Verification items for the finished model (mm, model axes). Face numbers are marked on the shaded views. A direction names the side the tool comes from. Round coordinates to 2 decimals unless told otherwise and drop trailing zeros. Write each loop counter-clockwise with the first axis right and the second up, starting at its lowest first coordinate (ties: lowest second). Pieces come first, ordered by that corner, then holes. Notation, with made-up numbers: M -14.75,15.5 L 19.25,15.5 A25 cw 19.25,43.5 Z; hole C 25,88.25 d6. An arc over 180 degrees is marked long. One line per question, with ' | ' between items.
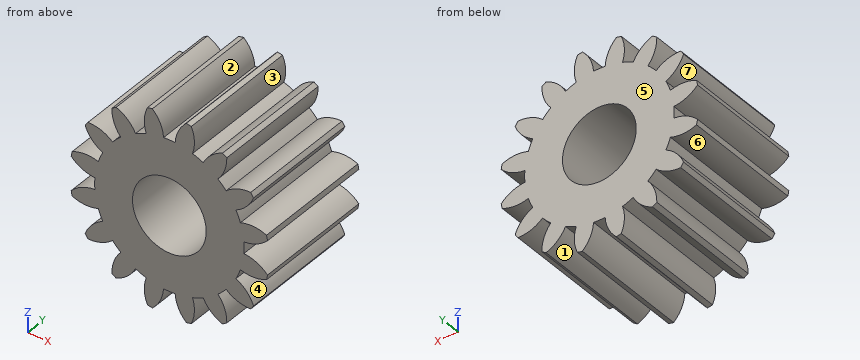
from build123d import *

# Parameters (mm, degrees)
BOSS_EXTRUDE1_DEPTH = 10
SKETCH2_R           = 3
CUT_EXTRUDE1_DEPTH  = 10


with BuildPart() as part:
    # Sketch1 → Boss-Extrude1 (new body)
    with BuildSketch(Plane(origin=(0, 0, 0), x_dir=(1, 0, 0), z_dir=(0, 1, 0))):
        with BuildLine():
            ThreePointArc((-7.982172642, 1.3765609), (-7.105660658, 0.739320543), (-6.05570223, 0.47111199))
            ThreePointArc((-6.05570223, 0.47111199), (-6.074, 0), (-6.05570223, -0.47111199))
            ThreePointArc((-6.05570223, -0.47111199), (-7.105660658, -0.739320543), (-7.982172642, -1.3765609))
            ThreePointArc((-7.982172642, -1.3765609), (-7.944360771, -1.580231608), (-7.901352979, -1.782868784))
            ThreePointArc((-7.901352979, -1.782868784), (-6.84770017, -2.036175492), (-5.775026098, -1.882166189))
            ThreePointArc((-5.775026098, -1.882166189), (-5.61164428, -2.324419168), (-5.414452591, -2.75266764))
            ThreePointArc((-5.414452591, -2.75266764), (-6.281848724, -3.402261728), (-6.847778879, -4.326421665))
            ThreePointArc((-6.847778879, -4.326421665), (-6.73490386, -4.500118887), (-6.617623951, -4.670872857))
            ThreePointArc((-6.617623951, -4.670872857), (-5.547239406, -4.501682267), (-4.615154594, -3.948901628))
            ThreePointArc((-4.615154594, -3.948901628), (-4.294966589, -4.294966589), (-3.948901628, -4.615154594))
            ThreePointArc((-3.948901628, -4.615154594), (-4.501682267, -5.547239406), (-4.670872857, -6.617623951))
            ThreePointArc((-4.670872857, -6.617623951), (-4.500118887, -6.73490386), (-4.326421665, -6.847778879))
            ThreePointArc((-4.326421665, -6.847778879), (-3.402261728, -6.281848724), (-2.75266764, -5.414452591))
            ThreePointArc((-2.75266764, -5.414452591), (-2.324419168, -5.61164428), (-1.882166189, -5.775026098))
            ThreePointArc((-1.882166189, -5.775026098), (-2.036175492, -6.84770017), (-1.782868784, -7.901352979))
            ThreePointArc((-1.782868784, -7.901352979), (-1.580231608, -7.944360771), (-1.3765609, -7.982172642))
            ThreePointArc((-1.3765609, -7.982172642), (-0.739320543, -7.105660658), (-0.47111199, -6.05570223))
            ThreePointArc((-0.47111199, -6.05570223), (0, -6.074), (0.47111199, -6.05570223))
            ThreePointArc((0.47111199, -6.05570223), (0.739320543, -7.105660658), (1.3765609, -7.982172642))
            ThreePointArc((1.3765609, -7.982172642), (1.580231608, -7.944360771), (1.782868784, -7.901352979))
            ThreePointArc((1.782868784, -7.901352979), (2.036175492, -6.84770017), (1.882166189, -5.775026098))
            ThreePointArc((1.882166189, -5.775026098), (2.324419168, -5.61164428), (2.75266764, -5.414452591))
            ThreePointArc((2.75266764, -5.414452591), (3.402261728, -6.281848724), (4.326421665, -6.847778879))
            ThreePointArc((4.326421665, -6.847778879), (4.500118887, -6.73490386), (4.670872857, -6.617623951))
            ThreePointArc((4.670872857, -6.617623951), (4.501682267, -5.547239406), (3.948901628, -4.615154594))
            ThreePointArc((3.948901628, -4.615154594), (4.294966589, -4.294966589), (4.615154594, -3.948901628))
            ThreePointArc((4.615154594, -3.948901628), (5.547239406, -4.501682267), (6.617623951, -4.670872857))
            ThreePointArc((6.617623951, -4.670872857), (6.73490386, -4.500118887), (6.847778879, -4.326421665))
            ThreePointArc((6.847778879, -4.326421665), (6.281848724, -3.402261728), (5.414452591, -2.75266764))
            ThreePointArc((5.414452591, -2.75266764), (5.61164428, -2.324419168), (5.775026098, -1.882166189))
            ThreePointArc((5.775026098, -1.882166189), (6.84770017, -2.036175492), (7.901352979, -1.782868784))
            ThreePointArc((7.901352979, -1.782868784), (7.944360771, -1.580231608), (7.982172642, -1.3765609))
            ThreePointArc((7.982172642, -1.3765609), (7.105660658, -0.739320543), (6.05570223, -0.47111199))
            ThreePointArc((6.05570223, -0.47111199), (6.074, 0), (6.05570223, 0.47111199))
            ThreePointArc((6.05570223, 0.47111199), (7.105660658, 0.739320543), (7.982172642, 1.3765609))
            ThreePointArc((7.982172642, 1.3765609), (7.944360771, 1.580231608), (7.901352979, 1.782868784))
            ThreePointArc((7.901352979, 1.782868784), (6.84770017, 2.036175492), (5.775026098, 1.882166189))
            ThreePointArc((5.775026098, 1.882166189), (5.61164428, 2.324419168), (5.414452591, 2.75266764))
            ThreePointArc((5.414452591, 2.75266764), (6.281848724, 3.402261728), (6.847778879, 4.326421665))
            ThreePointArc((6.847778879, 4.326421665), (6.73490386, 4.500118887), (6.617623951, 4.670872857))
            ThreePointArc((6.617623951, 4.670872857), (5.547239406, 4.501682267), (4.615154594, 3.948901628))
            ThreePointArc((4.615154594, 3.948901628), (4.294966589, 4.294966589), (3.948901628, 4.615154594))
            ThreePointArc((3.948901628, 4.615154594), (4.501682267, 5.547239406), (4.670872857, 6.617623951))
            ThreePointArc((4.670872857, 6.617623951), (4.500118887, 6.73490386), (4.326421665, 6.847778879))
            ThreePointArc((4.326421665, 6.847778879), (3.402261728, 6.281848724), (2.75266764, 5.414452591))
            ThreePointArc((2.75266764, 5.414452591), (2.324419168, 5.61164428), (1.882166189, 5.775026098))
            ThreePointArc((1.882166189, 5.775026098), (2.036175492, 6.84770017), (1.782868784, 7.901352979))
            ThreePointArc((1.782868784, 7.901352979), (1.580231608, 7.944360771), (1.3765609, 7.982172642))
            ThreePointArc((1.3765609, 7.982172642), (0.739320543, 7.105660658), (0.47111199, 6.05570223))
            ThreePointArc((0.47111199, 6.05570223), (0, 6.074), (-0.47111199, 6.05570223))
            ThreePointArc((-0.47111199, 6.05570223), (-0.739320543, 7.105660658), (-1.3765609, 7.982172642))
            ThreePointArc((-1.3765609, 7.982172642), (-1.580231608, 7.944360771), (-1.782868784, 7.901352979))
            ThreePointArc((-1.782868784, 7.901352979), (-2.036175492, 6.84770017), (-1.882166189, 5.775026098))
            ThreePointArc((-1.882166189, 5.775026098), (-2.324419168, 5.61164428), (-2.75266764, 5.414452591))
            ThreePointArc((-2.75266764, 5.414452591), (-3.402261728, 6.281848724), (-4.326421665, 6.847778879))
            ThreePointArc((-4.326421665, 6.847778879), (-4.500118887, 6.73490386), (-4.670872857, 6.617623951))
            ThreePointArc((-4.670872857, 6.617623951), (-4.501682267, 5.547239406), (-3.948901628, 4.615154594))
            ThreePointArc((-3.948901628, 4.615154594), (-4.294966589, 4.294966589), (-4.615154594, 3.948901628))
            ThreePointArc((-4.615154594, 3.948901628), (-5.547239406, 4.501682267), (-6.617623951, 4.670872857))
            ThreePointArc((-6.617623951, 4.670872857), (-6.73490386, 4.500118887), (-6.847778879, 4.326421665))
            ThreePointArc((-6.847778879, 4.326421665), (-6.281848724, 3.402261728), (-5.414452591, 2.75266764))
            ThreePointArc((-5.414452591, 2.75266764), (-5.61164428, 2.324419168), (-5.775026098, 1.882166189))
            ThreePointArc((-5.775026098, 1.882166189), (-6.84770017, 2.036175492), (-7.901352979, 1.782868784))
            ThreePointArc((-7.901352979, 1.782868784), (-7.944360771, 1.580231608), (-7.982172642, 1.3765609))
        make_face()
    extrude(amount=BOSS_EXTRUDE1_DEPTH)

    # Sketch2 → Cut-Extrude1 (cut)
    with BuildSketch(Plane(origin=(0, 10, 0), x_dir=(1, 0, 0), z_dir=(0, 1, 0))):
        Circle(SKETCH2_R)
    extrude(amount=-CUT_EXTRUDE1_DEPTH, mode=Mode.SUBTRACT)


solid = part.part
1. Section check A-A, the plane x = 0. Record the cut outline in (y, z), then the cut area to 3 significant figures.
Results:
outline: M 0,-6.07 L 10,-6.07 L 10,-3 L 0,-3 Z; M 0,3 L 10,3 L 10,6.07 L 0,6.07 Z | area: 61.5 mm2
2. Section check B-B, the plane z = 0. Record the cut outline in (x, y), then the cut area to 3 significant figures.
Results:
outline: M -6.07,0 L -3,0 L -3,10 L -6.07,10 Z; M 3,0 L 6.07,0 L 6.07,10 L 3,10 Z | area: 61.5 mm2
3. Go/stop test with flat-tipped pins: P1, Ø3, axis at y = 4.5, z = -5.5, coming from the -X side; P2, Ø1, axis at x = 4.5, y = 8.5, coming from the -Z side. Record where each tip stops, or that it passes through.
Results:
P1: stops at x = -6.85 | P2: stops at z = -6.85
4. Thickness scan on line 1 (Z direction, x = -4.25, y = 3.75); line 2 (X direction, y = 4.5, z = -0.75); line 3 (Z direction, x = -6.75, y = 7.25). Record the ranges inside material, lowest first.
Results:
line 1: z = -6.82 to -5.02, -4.34 to 4.34, 5.02 to 6.82 | line 2: x = -7.13 to -2.9, 2.9 to 7.13 | line 3: z = -4.48 to -4.1, -2.04 to -0.6, 0.6 to 2.04, 4.1 to 4.48
5. Mould release check, pull along X, two halves, no side actions. Record for the marked faces 4, 5, 6 and 7: pulls with the +X half, pulls with the -X half, needs draft (parallel to the pull), parting line crosses it, or undercut.
Results:
face 4: pulls with the +X half | face 5: needs draft | face 6: undercut | face 7: pulls with the -X half
6. Tool access check on the marked faces 1, 2 and 3. Record the directions out of +Z, -Z, +X, -X, +Y, -Y that give a thin tool (end or side, any length) a straight path to the whole face; none if there is none.
Results:
face 1: -Z, +Y, -Y | face 2: +Z, +Y, -Y | face 3: +Y, -Y
